Answer from the drawing. Dimensions are ordinates in mm from the lowest x, y and z of the part. A direction names the side the tool comes from. Give positions to 0.01 mm unless a question says otherwise; leave off trailing zeros. Write each loop counter-clockwise with the first axis right and the second up, starting at its lowest first coordinate (ties: lowest second). Pieces come first, ordered by that corner, then holes. Notation, with made-up numbers: (75.5, 15.5) -> (103.5, 15.5) arc R19 ccw to (103.5, 43.5) -> close; hole circle Ø1 at (-17, 16). An arc over 180 degrees is marked (long way). Write item = value, one per line.
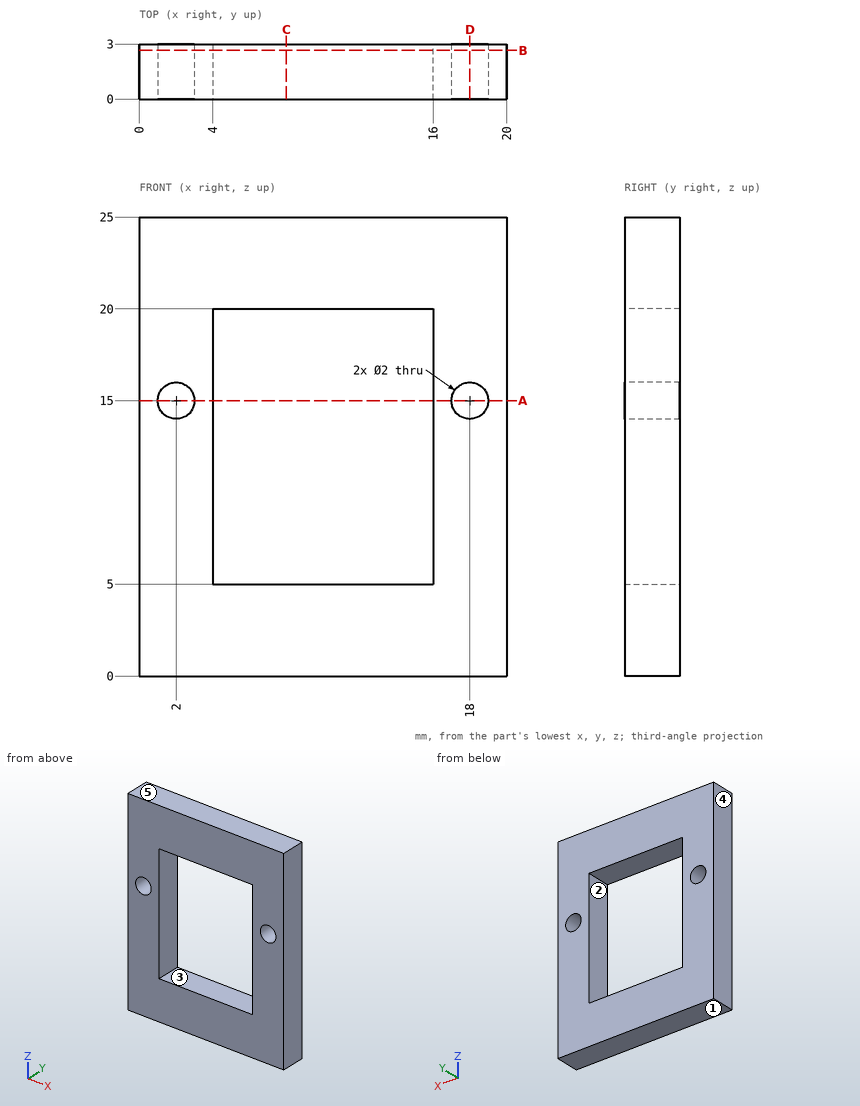
(1) Given P1, Ø8, axis at x = 16, z = 17, coming from the -Y side; P2, Ø1.6, axis at x = 18, z = 15, coming from the -Y side, each flat-ended and moving along its own axis, determine where each tip first touches the part or whether it passes through.
Checks:
P1 = 0
P2 = through
(2) Consider L1, parallel to X at y = 2.3, z = 15; L2, parallel to Z at x = 4.5, y = 1.3; L3, parallel to X at y = 1.95, z = 5.5. Determine where each line is inside the solid, lowest interval first.
Checks:
L1 = 0 to 1, 3 to 4, 16 to 17, 19 to 20
L2 = 0 to 5, 20 to 25
L3 = 0 to 4, 16 to 20
(3) The part is cut by section B-B on y = 2.65. Determine the outline of the cut face in (x, z), plus the area to 3 significant figures.
Checks:
outline = (0, 0) -> (20, 0) -> (20, 25) -> (0, 25) -> close; hole circle Ø2 at (2, 15); hole (4, 5) -> (16, 5) -> (16, 20) -> (4, 20) -> close; hole circle Ø2 at (18, 15)
area = 314 mm²
(4) For a pull along Z with two mould halves and no side action, classify the marked faces 3, 4 and 5 as released by +Z, released by -Z, zero draft, split by the parting line, or undercut.
Checks:
face_3 = undercut
face_4 = zero draft
face_5 = released by +Z
(5) The part is cut by section D-D on x = 18. Determine the outline of the cut face in (y, z).
Checks:
outline = (0, 0) -> (3, 0) -> (3, 14) -> (0, 14) -> close; (0, 16) -> (3, 16) -> (3, 25) -> (0, 25) -> close
(6) A tool of negligible diameter and unlimited length cuts with its end or side. For the marked faces 1 and 2, from which of +Z, -Z, +X, -X, +Y, -Y can it reach the whole face along a straight path? Write none if from no direction.
Checks:
face_1 = -Z, +X, -X, +Y, -Y
face_2 = +Y, -Y
(7) The part is cut by section C-C on x = 8. Determine the outline of the cut face in (y, z).
Checks:
outline = (0, 0) -> (3, 0) -> (3, 5) -> (0, 5) -> close; (0, 20) -> (3, 20) -> (3, 25) -> (0, 25) -> close
(8) The part is cut by section A-A on z = 15. Determine the outline of the cut face in (x, y).
Checks:
outline = (0, 0) -> (1, 0) -> (1, 3) -> (0, 3) -> close; (3, 0) -> (4, 0) -> (4, 3) -> (3, 3) -> close; (16, 0) -> (17, 0) -> (17, 3) -> (16, 3) -> close; (19, 0) -> (20, 0) -> (20, 3) -> (19, 3) -> close
